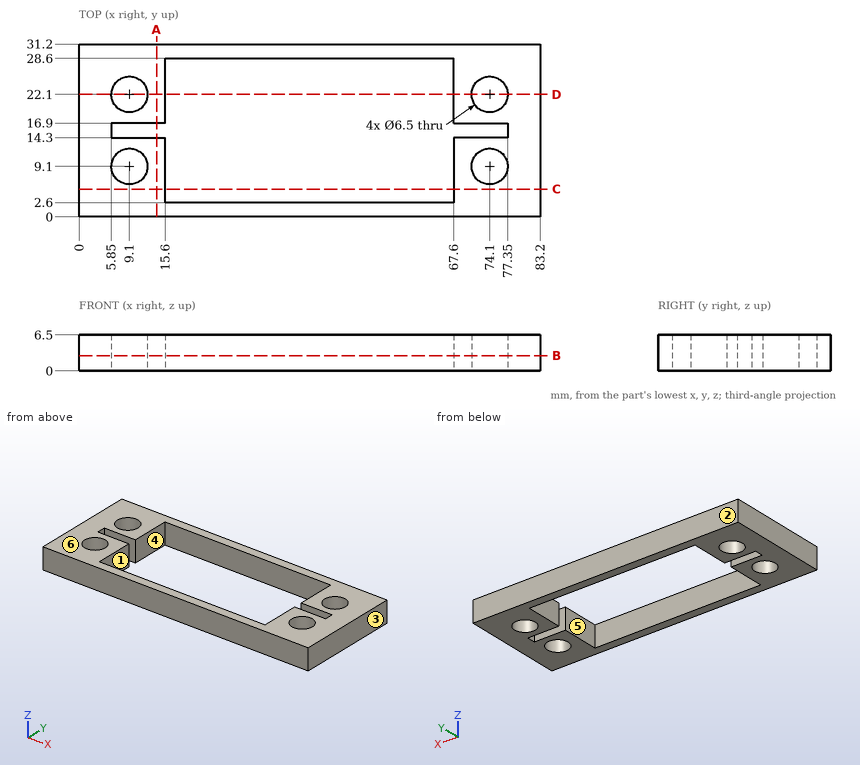
Drawing for the job (mm, zero at the part's lowest x, y, z). A direction names the side the tool comes from. Give positions to 0.01 mm unless a question says otherwise; leave off trailing zeros. Order: outer loops, then holes, each group sorted by start corner. A loop starts at its lowest first (then second) coordinate and runs counter-clockwise, first axis right, second up. Notation, with made-up numbers: M -37.75,77 L -30.75,77 A28 ccw -30.75,113 Z; hole C 61,-13 d1. An arc over 180 degrees is marked long. Use a Markdown table: item, result. Add a question column.
(1) 3-axis set-ups, long thin cutter, end or side, ignore diameter. For the marked faces 5 and 6: which of +Z, -Z, +X, -X, +Y, -Y reach the whole face in a straight line?
(2) Mould opens along X. For the marked faces 1, 2, 3 and 4 say: +X half, -X half, draft (parallel to the pull), parting line (faces both ways), or undercut.
(3) Saw through at D-D, the plane y = 22.1. Give the cut face in (x, z), and give its area (3 significant figures).
(4) Probe line 1 along X through (y, z) = (22.1, 3.25); line 2 along Y through (x, z) = (22, 5); line 3 along X through (y, z) = (6.5, 6). List the from-to ranges inside material, lowest first. Write a range as [from, to].
(5) Saw through at C-C, the plane y = 5. Give the cut face in (x, z).
(6) Saw through at A-A, the plane x = 14. Give the cut face in (y, z).
(7) Saw through at B-B, the plane z = 2.75. Give the cut face in (x, y).
Answer key:
| question | item | result |
|---|---|---|
| 1 | face 5 | +Z, -Z |
| 1 | face 6 | +Z, +X, -X, +Y, -Y |
| 2 | face 1 | undercut |
| 2 | face 2 | draft |
| 2 | face 3 | +X half |
| 2 | face 4 | undercut |
| 3 | outline | M 0,0 L 5.85,0 L 5.85,6.5 L 0,6.5 Z; M 12.35,0 L 15.6,0 L 15.6,6.5 L 12.35,6.5 Z; M 67.6,0 L 70.85,0 L 70.85,6.5 L 67.6,6.5 Z; M 77.35,0 L 83.2,0 L 83.2,6.5 L 77.35,6.5 Z |
| 3 | area | 118 mm^2 |
| 4 | line 1 | [0, 5.85], [12.35, 15.6], [67.6, 70.85], [77.35, 83.2] |
| 4 | line 2 | [0, 2.6], [28.6, 31.2] |
| 4 | line 3 | [0, 7.15], [11.05, 15.6], [67.6, 72.15], [76.05, 83.2] |
| 5 | outline | M 0,0 L 15.6,0 L 15.6,6.5 L 0,6.5 Z; M 67.6,0 L 83.2,0 L 83.2,6.5 L 67.6,6.5 Z |
| 6 | outline | M 0,0 L 14.3,0 L 14.3,6.5 L 0,6.5 Z; M 16.9,0 L 31.2,0 L 31.2,6.5 L 16.9,6.5 Z |
| 7 | outline | M 0,0 L 83.2,0 L 83.2,31.2 L 0,31.2 Z; hole C 9.1,9.1 d6.5; hole M 5.85,14.3 L 15.6,14.3 L 15.6,2.6 L 67.6,2.6 L 67.6,14.3 L 77.35,14.3 L 77.35,16.9 L 67.6,16.9 L 67.6,28.6 L 15.6,28.6 L 15.6,16.9 L 5.85,16.9 Z; hole C 9.1,22.1 d6.5; hole C 74.1,9.1 d6.5; hole C 74.1,22.1 d6.5 |
